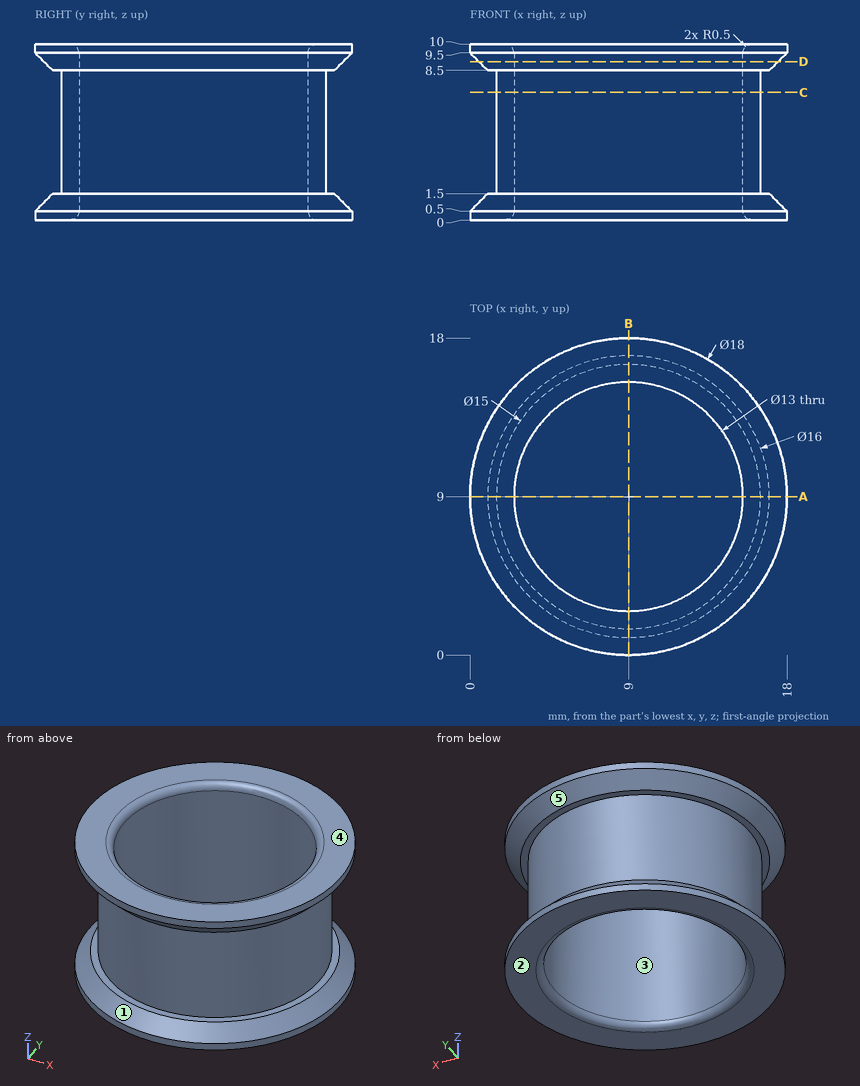
Print and shaded views of the part. All mm, measured from the part's lowest x, y and z. A direction names the side the tool comes from. Give positions to 0.01 mm unless a question says otherwise; leave off trailing zeros. Loops run counter-clockwise (first coordinate to the right, second up) from the corner with the lowest first, then second, coordinate; pieces in that order, holes last.
1) Saw through at A-A (y = 9). Write the cut outline in (x, z), plus the area to 3 significant figures.
2) Pull direction X, two halves, no side cores. Call the marked faces 1, 2 and 3: +X half, -X half, draft (parallel to the pull), parting line (faces both ways), or undercut.
3) Saw through at C-C (z = 7.25). Write the cut outline in (x, y).
4) Saw through at D-D (z = 9). Write the cut outline in (x, y).
5) Tool access for the marked faces 4 and 5: list every direction of +Z, -Z, +X, -X, +Y, -Y with a clear straight run to the whole face (end or side of a thin tool).
6) Flat gauge pins, fed straight in: pin 1 Ø1 at (x, z) = (8.5, 7.5) entering from +Y; pin 2 Ø8 at (x, y) = (8, 10.5) entering from +Z; pin 3 Ø6 at (x, z) = (2.5, 5) entering from -Y; pin 4 Ø5 at (x, z) = (9, 6.5) entering from +Y. Where does each tip first touch, or does it go through?
7) Wall check: line 1 (Y direction, x = 9, z = 4.5); line 2 (Z direction, x = 16, y = 12.5); line 3 (X direction, y = 13.5, z = 6). Give the ranges that are in metal, low to high.
Answer block:
1. outline: (0, 0) - (2, 0) arc R0.5 ccw to (2.5, 0.5) - (2.5, 9.5) arc R0.5 ccw to (2, 10) - (0, 10) - (0, 9.5) - (1, 8.5) - (1.5, 8.5) - (1.5, 1.5) - (1, 1.5) - (0, 0.5) - close; (15.5, 0.5) arc R0.5 ccw to (16, 0) - (18, 0) - (18, 0.5) - (17, 1.5) - (16.5, 1.5) - (16.5, 8.5) - (17, 8.5) - (18, 9.5) - (18, 10) - (16, 10) arc R0.5 ccw to (15.5, 9.5) - close
1. area: 26.8 mm2
2. face 1: parting line
2. face 2: draft
2. face 3: undercut
3. outline: circle Ø15 at (9, 9); hole circle Ø13 at (9, 9)
4. outline: circle Ø17 at (9, 9); hole circle Ø13 at (9, 9)
5. face 4: +Z, +X, -X, +Y, -Y
5. face 5: none
6. pin 1: stops at y = 16.5
6. pin 2: passes through
6. pin 3: stops at y = 2.37
6. pin 4: stops at y = 17.5
7. line 1: y = 1.5 to 2.5, 15.5 to 16.5
7. line 2: z = 0 to 1.5, 8.5 to 10
7. line 3: x = 3 to 4.31, 13.69 to 15
